from build123d import *

# Parameters (mm, degrees)
SKETCH1_W                = 12
SKETCH1_H                = 12
BOSS_EXTRUDE1_DEPTH      = 2
SKETCH2_W                = 54
SKETCH2_H                = 15
BOSS_EXTRUDE2_DEPTH      = 4
SKETCH3_W                = 12
SKETCH3_H                = 12
BOSS_EXTRUDE3_DEPTH      = 2
SKETCH4_R                = 1.5
CUT_EXTRUDE1_DEPTH       = 9
SKETCH5_W                = 10
SKETCH5_H                = 5
BOSS_EXTRUDE4_DEPTH      = 15
BOSS_EXTRUDE4_DEPTH_BACK = 5
SKETCH6_W                = 30
SKETCH6_H                = 20
BOSS_EXTRUDE5_DEPTH      = 3
SKETCH7_W                = 24
SKETCH7_H                = 4
CUT_EXTRUDE2_DEPTH       = 3


with BuildPart() as part:
    # Sketch1 → Boss-Extrude1 (new body)
    with BuildSketch(Plane.XY):
        with Locations((1.668449198, -3.417112299)):
            Rectangle(SKETCH1_W, SKETCH1_H)
    extrude(amount=BOSS_EXTRUDE1_DEPTH)

    # Sketch2 → Boss-Extrude2 (add)
    with BuildSketch(Plane(origin=(0, 0, 0), x_dir=(-1, 0, 0), z_dir=(0, 0, -1))):
        with Locations((-22.668449198, -1.917112299)):
            Rectangle(SKETCH2_W, SKETCH2_H)
    extrude(amount=BOSS_EXTRUDE2_DEPTH)

    # Sketch3 → Boss-Extrude3 (add)
    with BuildSketch(Plane.XY):
        with Locations((15.668449198, -3.417112299)):
            Rectangle(SKETCH3_W, SKETCH3_H)
        with Locations((29.668449198, -3.417112299)):
            Rectangle(SKETCH3_W, SKETCH3_H)
        with Locations((43.668449198, -3.417112299)):
            Rectangle(SKETCH3_W, SKETCH3_H)
    extrude(amount=BOSS_EXTRUDE3_DEPTH)

    # Sketch4 → Cut-Extrude1 (cut)
    with BuildSketch(Plane.XY.offset(2)):
        with Locations((1.668449198, -4.417112299)):
            Circle(SKETCH4_R)
        with Locations((15.668449198, -4.417112299)):
            Circle(SKETCH4_R)
        with Locations((29.668449198, -4.417112299)):
            Circle(SKETCH4_R)
        with Locations((43.668449198, -4.417112299)):
            Circle(SKETCH4_R)
    extrude(amount=-CUT_EXTRUDE1_DEPTH, mode=Mode.SUBTRACT)

    # Sketch5 → Boss-Extrude4 (add, two sides)
    with BuildSketch(Plane(origin=(0, 5.582887701, 0), x_dir=(1, 0, 0), z_dir=(0, 1, 0))) as boss_extrude4_sk:
        with Locations((22.668449198, 2.5)):
            Rectangle(SKETCH5_W, SKETCH5_H)
    extrude(amount=BOSS_EXTRUDE4_DEPTH)
    extrude(boss_extrude4_sk.sketch, amount=-BOSS_EXTRUDE4_DEPTH_BACK)

    # Sketch6 → Boss-Extrude5 (add)
    with BuildSketch(Plane(origin=(0, 20.582887701, 0), x_dir=(1, 0, 0), z_dir=(0, 1, 0))):
        with Locations((22.668449198, 10)):
            Rectangle(SKETCH6_W, SKETCH6_H)
    extrude(amount=BOSS_EXTRUDE5_DEPTH)

    # Sketch7 → Cut-Extrude2 (cut)
    with BuildSketch(Plane(origin=(0, 23.582887701, 0), x_dir=(1, 0, 0), z_dir=(0, 1, 0))):
        with Locations((22.668449198, 15)):
            Rectangle(SKETCH7_W, SKETCH7_H)
    extrude(amount=-CUT_EXTRUDE2_DEPTH, mode=Mode.SUBTRACT)


solid = part.part
Model file for the job. Use its own axes, mm. A direction names the side the tool comes from. Round coordinates to 2 decimals unless told otherwise and drop trailing zeros. Order: outer loops, then holes, each group sorted by start corner. A loop starts at its lowest first (then second) coordinate and runs counter-clockwise, first axis right, second up.
(1) Band-saw the part on A-A (x = 19). List the corners of the cut face in (y, z), then the cut area to 3 significant figures.
(2) Band-saw the part on B-B (z = -16). List the corners of the cut face in (x, y), then the cut area to 3 significant figures.
(3) Band-saw the part on C-C (y = 3.5). List the corners of the cut face in (x, z).
(4) 3-axis set-ups, long thin cutter, end or side, ignore diameter. For faces 1 (the face through (21.668, -4, 1)), 2 (the face through (30, 2.583, 1)), 3 (the face through (7, 5.583, -2)), 4 (the face through (10.668, 22, -15)): which of +Z, -Z, +X, -X, +Y, -Y reach the whole face in a straight line?
(5) Drill centre lines: line 1 (Y direction, x = 9.5, z = -1.75); line 2 (Z direction, x = 8, y = 22.5); line 3 (Z direction, x = 26, y = 19). Where is each one in solid material? Low to high.
(6) Band-saw the part on D-D (z = -3). List the corners of the cut face in (x, y), then the cut area to 3 significant figures.
(7) Pull direction Z, two halves, no side cores. Call faces 5 (the face through (34.668, 22, -15)), 6 (the face through (2, 2.583, 1)), 7 (the face through (22, 22, -20)): released by +Z, released by -Z, zero draft, split by the parting line, or undercut.
(8) Pin check, flat tips, straight feed: pin 1 (1.5 mm diameter, centred on x = 3, z = -5.5, fed in from -Y); pin 2 (1 mm diameter, centred on x = 16, z = 1, fed in from +Y); pin 3 (2.5 mm diameter, centred on y = 21.5, z = -14.5, fed in from +X); pin 4 (3 mm diameter, centred on y = 10.5, z = -6, fed in from +X). Stop position of each tip, or through.
Verdict:
1. outline: (-9.42, -4) - (0.58, -4) - (0.58, -5) - (20.58, -5) - (20.58, -13) - (23.58, -13) - (23.58, 0) - (2.58, 0) - (2.58, 2) - (-9.42, 2) - close; (20.58, -20) - (23.58, -20) - (23.58, -17) - (20.58, -17) - close
1. area: 212 mm2
2. outline: (7.67, 20.58) - (10.67, 20.58) - (10.67, 23.58) - (7.67, 23.58) - close; (34.67, 20.58) - (37.67, 20.58) - (37.67, 23.58) - (34.67, 23.58) - close
2. area: 18.0 mm2
3. outline: (-4.33, -4) - (17.67, -4) - (17.67, -5) - (27.67, -5) - (27.67, -4) - (49.67, -4) - (49.67, 0) - (-4.33, 0) - close
4. face 1: +Z, +Y, -Y
4. face 2: +Z, +X, -X, +Y
4. face 3: +Z, -Z, -X
4. face 4: +Y, -Y
5. line 1: y = -9.42 to 5.58, 20.58 to 23.58
5. line 2: z = -20 to 0
5. line 3: z = -5 to 0
6. outline: (-4.33, -9.42) - (49.67, -9.42) - (49.67, 5.58) - (27.67, 5.58) - (27.67, 20.58) - (37.67, 20.58) - (37.67, 23.58) - (7.67, 23.58) - (7.67, 20.58) - (17.67, 20.58) - (17.67, 5.58) - (-4.33, 5.58) - close; hole circle Ø3 at (1.67, -4.42); hole circle Ø3 at (15.67, -4.42); hole circle Ø3 at (29.67, -4.42); hole circle Ø3 at (43.67, -4.42)
6. area: 1,020 mm2
7. face 5: undercut
7. face 6: zero draft
7. face 7: released by -Z
8. pin 1: passes through
8. pin 2: stops at y = 2.58
8. pin 3: stops at x = 37.67
8. pin 4: stops at x = 27.67
